Verification items for the finished model (mm, model axes). A direction names the side the tool comes from. Round coordinates to 2 decimals unless told otherwise and drop trailing zeros.
from build123d import *

# Parameters (mm, degrees)
F1_DEPTH = 12.5
F2_W     = 5
F2_H     = 30
F2_H_2   = 540


with BuildPart() as f1:
    # F0 (on Top) → F1 (new body, symmetric)
    with BuildSketch(Plane.XY):
        with BuildLine():
            ThreePointArc((-631.5362024307, 76.3261139393), (-630.0717363367, 72.7905800334), (-626.5362024307, 71.3261139393))
            Line((-626.5362024307, 71.3261139393), (563.4637975693, 71.3261139393))
            ThreePointArc((563.4637975693, 71.3261139393), (566.9993314752, 72.7905800334), (568.4637975693, 76.3261139393))
            Line((568.4637975693, 76.3261139393), (568.4637975693, 766.3261139393))
            ThreePointArc((568.4637975693, 766.3261139393), (566.9993314752, 769.8616478452), (563.4637975693, 771.3261139393))
            Line((563.4637975693, 771.3261139393), (-626.5362024307, 771.3261139393))
            ThreePointArc((-626.5362024307, 771.3261139393), (-630.0717363367, 769.8616478452), (-631.5362024307, 766.3261139393))
            Line((-631.5362024307, 766.3261139393), (-631.5362024307, 76.3261139393))
        make_face()
        with BuildLine():
            ThreePointArc((-601.5362024307, 146.3261139393), (-600.0717363367, 149.8616478452), (-596.5362024307, 151.3261139393))
            Line((-596.5362024307, 151.3261139393), (-556.5362024307, 151.3261139393))
            ThreePointArc((-556.5362024307, 151.3261139393), (-553.0006685248, 149.8616478452), (-551.5362024307, 146.3261139393))
            Line((-551.5362024307, 146.3261139393), (-551.5362024307, 106.3261139393))
            ThreePointArc((-551.5362024307, 106.3261139393), (-553.0006685248, 102.7905800334), (-556.5362024307, 101.3261139393))
            Line((-556.5362024307, 101.3261139393), (-596.5362024307, 101.3261139393))
            ThreePointArc((-596.5362024307, 101.3261139393), (-600.0717363367, 102.7905800334), (-601.5362024307, 106.3261139393))
            Line((-601.5362024307, 106.3261139393), (-601.5362024307, 146.3261139393))
        make_face(mode=Mode.SUBTRACT)
        with BuildLine():
            ThreePointArc((488.4637975693, 146.3261139393), (489.9282636633, 149.8616478452), (493.4637975693, 151.3261139393))
            Line((493.4637975693, 151.3261139393), (533.4637975693, 151.3261139393))
            ThreePointArc((533.4637975693, 151.3261139393), (536.9993314752, 149.8616478452), (538.4637975693, 146.3261139393))
            Line((538.4637975693, 146.3261139393), (538.4637975693, 106.3261139393))
            ThreePointArc((538.4637975693, 106.3261139393), (536.9993314752, 102.7905800334), (533.4637975693, 101.3261139393))
            Line((533.4637975693, 101.3261139393), (493.4637975693, 101.3261139393))
            ThreePointArc((493.4637975693, 101.3261139393), (489.9282636633, 102.7905800334), (488.4637975693, 106.3261139393))
            Line((488.4637975693, 106.3261139393), (488.4637975693, 146.3261139393))
        make_face(mode=Mode.SUBTRACT)
        with BuildLine():
            ThreePointArc((-601.5362024307, 736.3261139393), (-600.0717363367, 739.8616478452), (-596.5362024307, 741.3261139393))
            Line((-596.5362024307, 741.3261139393), (-556.5362024307, 741.3261139393))
            ThreePointArc((-556.5362024307, 741.3261139393), (-553.0006685248, 739.8616478452), (-551.5362024307, 736.3261139393))
            Line((-551.5362024307, 736.3261139393), (-551.5362024307, 696.3261139393))
            ThreePointArc((-551.5362024307, 696.3261139393), (-553.0006685248, 692.7905800334), (-556.5362024307, 691.3261139393))
            Line((-556.5362024307, 691.3261139393), (-596.5362024307, 691.3261139393))
            ThreePointArc((-596.5362024307, 691.3261139393), (-600.0717363367, 692.7905800334), (-601.5362024307, 696.3261139393))
            Line((-601.5362024307, 696.3261139393), (-601.5362024307, 736.3261139393))
        make_face(mode=Mode.SUBTRACT)
        with BuildLine():
            ThreePointArc((488.4637975693, 736.3261139393), (489.9282636633, 739.8616478452), (493.4637975693, 741.3261139393))
            Line((493.4637975693, 741.3261139393), (533.4637975693, 741.3261139393))
            ThreePointArc((533.4637975693, 741.3261139393), (536.9993314752, 739.8616478452), (538.4637975693, 736.3261139393))
            Line((538.4637975693, 736.3261139393), (538.4637975693, 696.3261139393))
            ThreePointArc((538.4637975693, 696.3261139393), (536.9993314752, 692.7905800334), (533.4637975693, 691.3261139393))
            Line((533.4637975693, 691.3261139393), (493.4637975693, 691.3261139393))
            ThreePointArc((493.4637975693, 691.3261139393), (489.9282636633, 692.7905800334), (488.4637975693, 696.3261139393))
            Line((488.4637975693, 696.3261139393), (488.4637975693, 736.3261139393))
        make_face(mode=Mode.SUBTRACT)
    extrude(amount=F1_DEPTH, both=True)

    # F2 (on face) → F3 (revolve, cut)
    with BuildSketch(Plane(origin=(0, 0, -12.5), x_dir=(1, 0, 0), z_dir=(0, 0, -1))):
        with Locations((-574.0362024307, -86.3261139393)):
            Rectangle(F2_W, F2_H)
        with Locations((-574.0362024307, -421.3261139393)):
            Rectangle(F2_W, F2_H_2)
        with Locations((-574.0362024307, -756.3261139393)):
            Rectangle(F2_W, F2_H)
    revolve(axis=Axis((-576.5362024307, 421.3261139393, -12.5), (0, -1, 0)), mode=Mode.SUBTRACT)


solid = f1.part
1. Release check for a two-part mould opening along X. For faces 1 (the face through (-40, 426, 12.5)), 2 (the face through (568.464, 416, 0)), 3 (the face through (-577, 151.326, 0)) record: released by +X, released by -X, zero draft, split by the parting line, or undercut.
2. Scan lines: L1, parallel to X at y = 700.5, z = -7.5; L2, parallel to Y at x = 489, z = -2.5; L3, parallel to X at y = 670, z = -8.5. Record each from-to range of solid material in increasing order.
3. Tool access check on faces 4 (the face through (514, 101.326, 0)), 5 (the face through (-631.536, 426, 0)). Record the directions out of +Z, -Z, +X, -X, +Y, -Y that give a thin tool (end or side, any length) a straight path to the whole face; none if there is none.
Taken from the geometry:
1. face 1: zero draft
1. face 2: released by +X
1. face 3: undercut
2. L1: x = -631.54 to -601.54, -551.54 to 488.46, 538.46 to 568.46
2. L2: y = 71.33 to 104.07, 148.58 to 694.07, 738.58 to 771.33
2. L3: x = -631.54 to -579.54, -573.54 to 568.46
3. face 4: +Z, -Z
3. face 5: +Z, -Z, -X, +Y, -Y
